```python
from build123d import *

# Parameters (mm, degrees)
CYLINDER002_R          = 3
CYLINDER002_DEPTH      = 2.5
CYLINDER004_R          = 1
CYLINDER004_DEPTH      = 8.5
CYLINDER003_R          = 1
CYLINDER003_DEPTH      = 8.5
CYLINDER_R             = 8
CYLINDER_DEPTH         = 34
CYLINDER001_R          = 1.5
CYLINDER001_DEPTH      = 8
FUSION_PLACEMENT_ANGLE = 44.999934


with BuildPart() as bearing:
    # Cylinder002 → Cylinder002 (new body)
    with BuildSketch(Plane.XY.offset(-2)):
        Circle(CYLINDER002_R)
    extrude(amount=CYLINDER002_DEPTH)


with BuildPart() as cylinder004:
    # Cylinder004 → Cylinder004 (new body)
    with BuildSketch(Plane(origin=(-5.5, 0, -8), x_dir=(1, 0, 0), z_dir=(0, 0, 1))):
        Circle(CYLINDER004_R)
    extrude(amount=CYLINDER004_DEPTH)


with BuildPart() as cylinder003:
    # Cylinder003 → Cylinder003 (new body)
    with BuildSketch(Plane(origin=(5.5, 0, -8), x_dir=(1, 0, 0), z_dir=(0, 0, 1))):
        Circle(CYLINDER003_R)
    extrude(amount=CYLINDER003_DEPTH)


with BuildPart() as cut001:
    # Cylinder → Cylinder (new body)
    with BuildSketch(Plane.XY):
        Circle(CYLINDER_R)
    extrude(amount=CYLINDER_DEPTH)

    # Cut: cut Cylinder003
    add(cylinder003.part, mode=Mode.SUBTRACT)

    # Cut001: cut Cylinder004
    add(cylinder004.part, mode=Mode.SUBTRACT)


with BuildPart() as obj1:
    # Cylinder001 → Cylinder001 (new body)
    with BuildSketch(Plane.XY.offset(-8)):
        Circle(CYLINDER001_R)
    extrude(amount=CYLINDER001_DEPTH)

    # Fusion: union bearing, Cut001
    add(bearing.part)
    add(cut001.part)


with BuildPart() as obj1_1:
    # Fusion placement: moved
    add(obj1.part.rotate(Axis((0, 0, 0), (0, 0, 1)), FUSION_PLACEMENT_ANGLE))


solid = obj1_1.part
```
Check sheet for the modelled part. Datum: model origin and axes. Units: mm. A direction names the side the tool comes from. Round coordinates to 2 decimals unless told otherwise and drop trailing zeros. Order: outer loops, then holes, each group sorted by start corner. A loop starts at its lowest first (then second) coordinate and runs counter-clockwise, first axis right, second up. Notation, with made-up numbers: (2.25, 26.5) - (39.25, 26.5) arc R27 cw to (39.25, 63.5) - close; hole circle Ø6 at (-31.5, 21). An arc over 180 degrees is marked (long way). Answer as CSV lines item,"result". Start each with the question number.
1) Depth check by flat-ended pin: pin 1 (4 mm diameter, centred on y = 3, z = 12.5, fed in from +X); pin 2 (3 mm diameter, centred on x = -4.5, z = 19, fed in from -Y); pin 3 (2 mm diameter, centred on x = 3.5, y = 4, fed in from -Z). Enter the tip coordinate at first touch or a pass-through.
2) Section check C-C (z = 30). Record the cut outline in (x, y).
3) Tool access check on faces 1 (the face through (4.351, 4.776, 0.246)), 2 (the face through (4.296, -6.749, 16.762)). Record the directions out of +Z, -Z, +X, -X, +Y, -Y that give a thin tool (end or side, any length) a straight path to the whole face; none if there is none.
4) Section check A-A (y = 0). Record the cut outline in (x, z), then the cut area to 3 significant figures.
5) Section check D-D (y = -4.5). Record the cut outline in (x, z), then the cut area to 3 significant figures.
6) Scan lines: probe 1 along Z at (x, y) = (6.5, -1); probe 2 along Z at (x, y) = (-1.5, -0.5); probe 3 along X at (y, z) = (-0.25, 18.5). Record each from-to range of solid material in increasing order.
7) Draft check along X on faces 3 (the face through (-0.196, -1.487, -5.042)), 4 (the face through (-4, -4, 0.5)), 5 (the face through (0, 0, -8)). Enter one of: +X half, -X half, draft (parallel to the pull), parting line (faces both ways), or undercut.
Determined:
1,pin 1,"x = 7.94"
1,pin 2,"y = -7.42"
1,pin 3,"z = 0"
2,outline,"circle Ø16 at (0, 0)"
3,face 1,"-Z"
3,face 2,"+Z, -Z"
4,outline,"(-8, 0) - (-3, 0) - (-3, -2) - (-1.5, -2) - (-1.5, -8) - (1.5, -8) - (1.5, -2) - (3, -2) - (3, 0) - (8, 0) - (8, 34) - (-8, 34) - close"
4,area,"574 mm^2"
5,outline,"(-6.61, 0) - (-4.68, 0) - (-4.68, 0.5) - (-3.1, 0.5) - (-3.1, 0) - (6.61, 0) - (6.61, 34) - (-6.61, 34) - close"
5,area,"449 mm^2"
6,probe 1,"0 to 34"
6,probe 2,"-2 to 34"
6,probe 3,"-8 to 8"
7,face 3,"parting line"
7,face 4,"undercut"
7,face 5,"draft"
